from build123d import *

# Parameters (mm, degrees)
BOSS_EXTRUDE1_DEPTH     = 75
CUT_EXTRUDE1_DEPTH      = 159.902485821
CUT_EXTRUDE1_DEPTH_BACK = 159.902485821
CUT_EXTRUDE2_DEPTH      = 159.902485821
CUT_EXTRUDE2_DEPTH_BACK = 159.902485821
BOSS_EXTRUDE3_START     = 115
BOSS_EXTRUDE3_DEPTH     = 2
BOSS_EXTRUDE5_START     = -115
BOSS_EXTRUDE5_DEPTH     = 2
FILLET3_R               = 5
FILLET4_R               = 20
FILLET5_R               = 10
FILLET6_R               = 10
FILLET7_R               = 10
FILLET8_R               = 10
FILLET11_R              = 1
BOSS_EXTRUDE6_REACH     = 266.055
SKETCH7_W               = 79.88
SKETCH7_H               = 51.8
FILLET13_R              = 5


with BuildPart() as part:
    # Sketch2 → Boss-Extrude1 (new body)
    with BuildSketch(Plane.XY):
        Polygon((-115, -60.3), (-65.9, -80), (65.9, -80), (115, -60.3), (115, 80), (-115, 80), align=None)
    extrude(amount=-BOSS_EXTRUDE1_DEPTH)

    # Sketch3 → Cut-Extrude1 (cut, two sides: drawn at the far end of the back side and taken through both)
    with BuildSketch(Plane(origin=(0, 0, 0), x_dir=(0, 0, -1), z_dir=(1, 0, 0)).offset(-CUT_EXTRUDE1_DEPTH_BACK)):
        Polygon((0, -80), (75, -38.15), (75, -80), align=None)
    extrude(amount=CUT_EXTRUDE1_DEPTH + CUT_EXTRUDE1_DEPTH_BACK, mode=Mode.SUBTRACT)

    # Sketch4 → Cut-Extrude2 (cut, two sides: drawn at the far end of the back side and taken through both)
    with BuildSketch(Plane(origin=(0, 0, 0), x_dir=(1, 0, 0), z_dir=(0, 1, 0)).offset(-CUT_EXTRUDE2_DEPTH_BACK)):
        Polygon((-115, 20.6), (-103, 0), (-115, 0), align=None)
        Polygon((115, 20.6), (103, 0), (115, 0), align=None)
    extrude(amount=CUT_EXTRUDE2_DEPTH + CUT_EXTRUDE2_DEPTH_BACK, mode=Mode.SUBTRACT)

    # Sketch5 → Boss-Extrude3 (add)
    with BuildSketch(Plane(origin=(0, 0, 0), x_dir=(0, 0, -1), z_dir=(1, 0, 0)).offset(BOSS_EXTRUDE3_START)):
        Polygon((30.6, -62.9252), (88.18, -38.439520512), (171.03, 87.993161576), (74.11, 87.993161576), (45, 33.512515472), align=None)
    extrude(amount=BOSS_EXTRUDE3_DEPTH)

    # Sketch6 → Boss-Extrude5 (add)
    with BuildSketch(Plane(origin=(0, 0, 0), x_dir=(0, 0, -1), z_dir=(1, 0, 0)).offset(BOSS_EXTRUDE5_START)):
        Polygon((30.6, -62.9252), (88.18, -38.439520512), (171.03, 87.993161576), (74.11, 87.993161576), (45, 33.512515472), align=None)
    extrude(amount=-BOSS_EXTRUDE5_DEPTH)

    # Fillet3
    fillet3_edges = [part.edges().sort_by_distance(p)[0] for p in [
        (116, 87.993161576, -171.03),
        (-116, 87.993161576, -171.03),
    ]]
    fillet(fillet3_edges, radius=FILLET3_R)

    # Fillet4
    # the kernel refuses this fillet: 20 mm, written as the material it takes off along each edge
    with BuildSketch(Plane(origin=(115, 87.993161576, -74.11), x_dir=(0, -0.8819920042873963, 0.4712643678160927), z_dir=(1, 0, 0)), Plane(origin=(-115, 87.993161576, -74.11), x_dir=(0, 0, -1), z_dir=(-1, 0, 0))) as fillet4_piece_1:
        with BuildLine():
            CenterArc((FILLET4_R * 0.599478940414, FILLET4_R), FILLET4_R, 208.116400727, 61.883599273)
            Line((-FILLET4_R * 0.282513063873, FILLET4_R * 0.528735632184), (0, 0))
            Line((0, 0), (FILLET4_R * 0.599478940414, 0))
        make_face()
    extrude(amount=31.973947021, mode=Mode.SUBTRACT)

    # Fillet5
    fillet5_edges = [part.edges().sort_by_distance(p)[0] for p in [
        (116, 33.512515472, -45),
    ]]
    fillet(fillet5_edges, radius=FILLET5_R)

    # Fillet6
    fillet6_edges = [part.edges().sort_by_distance(p)[0] for p in [
        (-116, -38.439520512, -88.18),
    ]]
    fillet(fillet6_edges, radius=FILLET6_R)

    # Fillet7
    fillet7_edges = [part.edges().sort_by_distance(p)[0] for p in [
        (-116, 33.512515472, -45),
    ]]
    fillet(fillet7_edges, radius=FILLET7_R)

    # Fillet8
    fillet8_edges = [part.edges().sort_by_distance(p)[0] for p in [
        (116, -38.439520512, -88.18),
    ]]
    fillet(fillet8_edges, radius=FILLET8_R)

    # Fillet11
    fillet11_edges = [part.edges().sort_by_distance(p)[0] for p in [
        (116, -62.9252, -30.6),
        (-116, -62.9252, -30.6),
    ]]
    fillet(fillet11_edges, radius=FILLET11_R)

    # Sketch7 → Boss-Extrude6 (add, up to next)
    with BuildSketch(Plane(origin=(0, -80, 0), x_dir=(-1, 0, 0), z_dir=(0, -1, 0)), mode=Mode.PRIVATE) as boss_extrude6_sk1:
        with Locations((0, 25.9)):
            Rectangle(SKETCH7_W, SKETCH7_H)
    boss_extrude6_tool1 = extrude(boss_extrude6_sk1.sketch, amount=-BOSS_EXTRUDE6_REACH, mode=Mode.PRIVATE) - part.part
    add(boss_extrude6_tool1.solids().sort_by_distance((0, -80, -25.9))[0])

    # Fillet13
    fillet13_edges = [part.edges().sort_by_distance(p)[0] for p in [
        (39.94, -65.5478, -51.8),
        (-39.94, -65.5478, -51.8),
    ]]
    fillet(fillet13_edges, radius=FILLET13_R)


solid = part.part
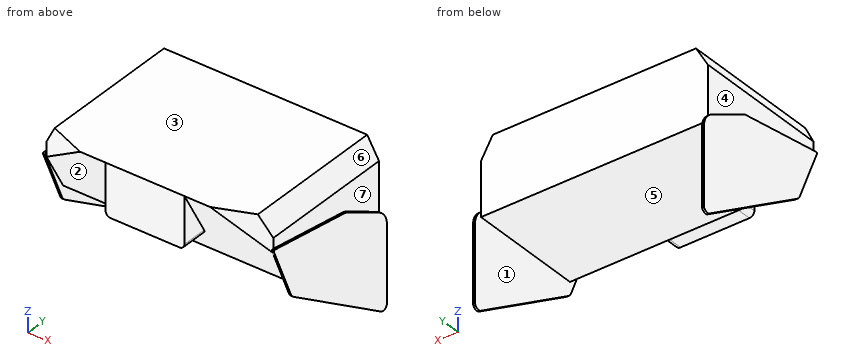
Check sheet for the modelled part. Datum: model origin and axes. Units: mm. Face numbers are marked on the shaded views. A direction names the side the tool comes from. Round coordinates to 2 decimals unless told otherwise and drop trailing zeros. Write each loop counter-clockwise with the first axis right and the second up, starting at its lowest first coordinate (ties: lowest second). Pieces come first, ordered by that corner, then holes. Notation, with made-up numbers: (-27, 23.25) - (10, 23.25) arc R30 ccw to (10, 51.25) - close; hole circle Ø3 at (86.5, -18). An arc over 180 degrees is marked (long way). Return JSON: item names as keys, results as strings.
Q1. Cross-section at D-D (z = -128). Record the boundary of the cut face in (x, y).
Returned:
{"outline": "(-117, 22.33) - (-115, 22.33) - (-115, 87.99) - (-117, 87.99) - close; (115, 22.33) - (117, 22.33) - (117, 87.99) - (115, 87.99) - close"}
Q2. Cross-section at A-A (z = -111). Record the boundary of the cut face in (x, y).
Returned:
{"outline": "(-117, -3.62) - (-115, -3.62) - (-115, 87.99) - (-117, 87.99) - close; (115, -3.62) - (117, -3.62) - (117, 87.99) - (115, 87.99) - close"}
Q3. Draft check along X on the marked faces 1, 2, 3 and 4. Enter one of: released by +X, released by -X, zero draft, split by the parting line, or undercut.
Returned:
{"face 1": "undercut", "face 2": "undercut", "face 3": "zero draft", "face 4": "released by -X"}
Q4. Cross-section at C-C (y = 56.5). Record the boundary of the cut face in (x, z), then the cut area to 3 significant figures.
Returned:
{"outline": "(-117, -150.39) - (-115, -150.39) - (-115, -75) - (115, -75) - (115, -150.39) - (117, -150.39) - (117, -57.28) - (115, -57.28) - (115, -20.6) - (103, 0) - (-103, 0) - (-115, -20.6) - (-115, -57.28) - (-117, -57.28) - close", "area": "17,400 mm²"}
Q5. Depth check by flat-ended pin: P1, Ø8.5, axis at x = 15.5, y = -66.5, coming from the -Z side; P2, Ø4, axis at y = 46.5, z = -28.5, coming from the -X side; P3, Ø4, axis at x = 11.5, y = -9.5, coming from the +Z side; P4, Ø5, axis at x = 54.5, z = -78, coming from the -Y side. Enter the tip coordinate at first touch or a pass-through.
Returned:
{"P1": "stops at z = -51.8", "P2": "stops at x = -115", "P3": "stops at z = 0", "P4": "passes through"}
Q6. Scan lines: L1, parallel to X at y = 48.5, z = -100.5; L2, parallel to Z at x = 81.5, y = 7.5; L3, parallel to X at y = -22, z = -36. Record each from-to range of solid material in increasing order. Write a range as from..to.
Returned:
{"L1": "x = -117..-115, 115..117", "L2": "z = -75..0", "L3": "x = -115..115"}
Q7. Access from +Z, -Z, +X, -X, +Y, -Y to the whole of each face (thin tool, end or side, straight path). Record for the marked faces 5, 6 and 7.
Returned:
{"face 5": "-Z, +Y, -Y", "face 6": "+Z, +X, +Y, -Y", "face 7": "+Z, +X, +Y"}
Q8. Cross-section at B-B (x = 29). Record the boundary of the cut face in (y, z), then the cut area to 3 significant figures.
Returned:
{"outline": "(-80, -51.8) - (-51.1, -51.8) - (-38.15, -75) - (80, -75) - (80, 0) - (-80, 0) - close", "area": "11,200 mm²"}
